Geometry: final body of the model. Coordinates: model frame, mm. Face numbers are marked on the shaded views. A direction names the side the tool comes from. Round coordinates to 2 decimals unless told otherwise and drop trailing zeros. Order: outer loops, then holes, each group sorted by start corner. A loop starts at its lowest first (then second) coordinate and runs counter-clockwise, first axis right, second up. Notation, with made-up numbers: M -11.5,8 L 24.5,8 A20 cw 24.5,31 Z; hole C 7,27.5 d10. An arc over 180 degrees is marked long. Put each result on its own line as item: value. Start each with the question number.
1) Draft query along Y for the marked faces 1, 2 and 3. Return one class per face: pulls with the +Y half, pulls with the -Y half, needs draft (parallel to the pull), parting line crosses it, or undercut.
2) Access query for the marked faces 4, 5 and 6. Directions: +Z, -Z, +X, -X, +Y, -Y. A direction counts if a zero-diameter tool reaches every point of the face in a straight line with its end or side. Return the directions, or none.
3) First-contact query: P1, Ø4, axis at x = 49.5, z = -11.5, coming from the +Y side; P2, Ø12, axis at x = 51, y = 10.5, coming from the -Z side; P3, Ø8, axis at x = 58.5, y = 28, coming from the +Z side. Flat tips, straight axial feed; report the tip coordinate or a pass-through.
4) Section A-A, the plane y = 54.5. Return loops of the section in (x, z), then the cut area to 3 significant figures.
5) Material intervals for probe 1 along Y at (x, z) = (56, 7); probe 2 along X at (y, z) = (35.5, -13.5); probe 3 along X at (y, z) = (47, 8.25), sorted ascending. Write a range as [from, to].
6) Section B-B, the plane x = 32. Return loops of the section in (y, z).
7) Section C-C, the plane z = -2. Return loops of the section in (x, y).
8) Section D-D, the plane y = 31.5. Return loops of the section in (x, z), then the cut area to 3 significant figures.
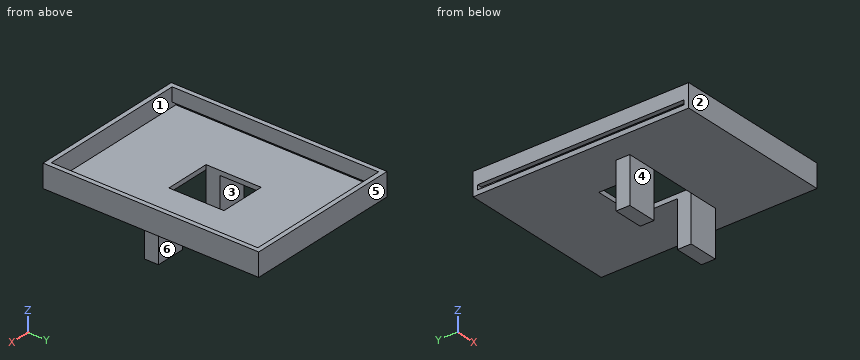
from build123d import *

# Parameters (mm, degrees)
SKETCH_W             = 69
SKETCH_H             = 94
SKETCH_W_2           = 65
SKETCH_H_2           = 90
PAD_DEPTH            = 10
SKETCH001_W          = 65
SKETCH001_H          = 90
PAD001_DEPTH         = 2
SKETCH002_W          = 90
SKETCH002_H          = 2
POCKET_DEPTH         = 2.001
SKETCH003_W          = 20
SKETCH003_H          = 24
POCKET001_DEPTH      = 0.001
POCKET001_DEPTH_BACK = -10.001
SKETCH004_W          = 13
SKETCH004_H          = 6
PAD002_DEPTH         = 20


with BuildPart() as part:
    # Sketch → Pad (new body)
    with BuildSketch(Plane.XY):
        with Locations((32.5, 45)):
            Rectangle(SKETCH_W, SKETCH_H)
        with Locations((32.5, 45)):
            Rectangle(SKETCH_W_2, SKETCH_H_2, mode=Mode.SUBTRACT)
    extrude(amount=PAD_DEPTH)

    # Sketch001 → Pad001 (join)
    with BuildSketch(Plane.XY):
        with Locations((32.5, 45)):
            Rectangle(SKETCH001_W, SKETCH001_H)
    extrude(amount=PAD001_DEPTH)

    # Sketch002 → Pocket (cut, through all)
    with BuildSketch(Plane.YZ):
        with Locations((45, 3)):
            Rectangle(SKETCH002_W, SKETCH002_H)
    extrude(amount=-POCKET_DEPTH, mode=Mode.SUBTRACT)

    # Sketch003 → Pocket001 (cut, two sides)
    with BuildSketch(Plane.XY) as pocket001_sk:
        with Locations((32.5, 45)):
            Rectangle(SKETCH003_W, SKETCH003_H)
    extrude(amount=-POCKET001_DEPTH, mode=Mode.SUBTRACT)
    extrude(pocket001_sk.sketch, amount=-POCKET001_DEPTH_BACK, mode=Mode.SUBTRACT)

    # Sketch004 → Pad002 (join)
    with BuildSketch(Plane.XY):
        with Locations((16, 36)):
            Rectangle(SKETCH004_W, SKETCH004_H)
        with Locations((49, 36)):
            Rectangle(SKETCH004_W, SKETCH004_H)
    extrude(amount=-PAD002_DEPTH)


solid = part.part
Result sheet:
1. face 1: undercut
1. face 2: pulls with the -Y half
1. face 3: pulls with the +Y half
2. face 4: -Z, +X, -X, -Y
2. face 5: +Z, -Z, +X, -X, +Y
2. face 6: -Z, +X, -X, +Y
3. P1: stops at y = 39
3. P2: stops at z = 0
3. P3: stops at z = 2
4. outline: M -2,0 L 22.5,0 L 22.5,2 L -2,2 Z; M -2,4 L 0,4 L 0,10 L -2,10 Z; M 42.5,0 L 67,0 L 67,10 L 65,10 L 65,2 L 42.5,2 Z
4. area: 126 mm2
5. probe 1: y = [-2, 0], [90, 92]
5. probe 2: x = [9.5, 22.5], [42.5, 55.5]
5. probe 3: x = [-2, 0], [65, 67]
6. outline: M -2,0 L 33,0 L 33,2 L 0,2 L 0,10 L -2,10 Z; M 57,0 L 92,0 L 92,10 L 90,10 L 90,2 L 57,2 Z
7. outline: M 9.5,33 L 22.5,33 L 22.5,39 L 9.5,39 Z; M 42.5,33 L 55.5,33 L 55.5,39 L 42.5,39 Z
8. outline: M -2,0 L 67,0 L 67,10 L 65,10 L 65,2 L -2,2 Z; M -2,4 L 0,4 L 0,10 L -2,10 Z
8. area: 166 mm2
